```python
from build123d import *

# Parameters (mm, degrees)
SKETCH1_W           = 48.3
SKETCH1_H           = 45
SKETCH1_R           = 2.875
SKETCH1_R_2         = 1.25
SKETCH1_R_3         = 2.8
SKETCH1_R_4         = 2.5
BOSS_EXTRUDE1_DEPTH = 6.35


with BuildPart() as part:
    # Sketch1 → Boss-Extrude1 (new body)
    with BuildSketch(Plane(origin=(0, 0, 0), x_dir=(1, 0, 0), z_dir=(0, 1, 0))):
        with Locations((24.15, -22.5)):
            Rectangle(SKETCH1_W, SKETCH1_H)
        with Locations(Location((15.8, -12.5, 0), (0, 0, 270))):
            Circle(SKETCH1_R, mode=Mode.SUBTRACT)
        with Locations(Location((35.8, -12.5, 0), (0, 0, 270))):
            Circle(SKETCH1_R, mode=Mode.SUBTRACT)
        with Locations(Location((15.8, -32.5, 0), (0, 0, 270))):
            Circle(SKETCH1_R, mode=Mode.SUBTRACT)
        with Locations(Location((35.8, -32.5, 0), (0, 0, 270))):
            Circle(SKETCH1_R, mode=Mode.SUBTRACT)
        with Locations(Location((10.8, -7, 0), (0, 0, 270))):
            Circle(SKETCH1_R_2, mode=Mode.SUBTRACT)
        with Locations(Location((20.8, -7, 0), (0, 0, 270))):
            Circle(SKETCH1_R_2, mode=Mode.SUBTRACT)
        with Locations(Location((30.8, -7, 0), (0, 0, 270))):
            Circle(SKETCH1_R_2, mode=Mode.SUBTRACT)
        with Locations(Location((40.8, -7, 0), (0, 0, 270))):
            Circle(SKETCH1_R_2, mode=Mode.SUBTRACT)
        with Locations(Location((20.8, -17, 0), (0, 0, 270))):
            Circle(SKETCH1_R_2, mode=Mode.SUBTRACT)
        with Locations(Location((30.8, -17, 0), (0, 0, 270))):
            Circle(SKETCH1_R_2, mode=Mode.SUBTRACT)
        with Locations(Location((40.8, -17, 0), (0, 0, 270))):
            Circle(SKETCH1_R_2, mode=Mode.SUBTRACT)
        with Locations(Location((20.8, -27, 0), (0, 0, 270))):
            Circle(SKETCH1_R_2, mode=Mode.SUBTRACT)
        with Locations(Location((30.8, -27, 0), (0, 0, 270))):
            Circle(SKETCH1_R_2, mode=Mode.SUBTRACT)
        with Locations(Location((40.8, -27, 0), (0, 0, 270))):
            Circle(SKETCH1_R_2, mode=Mode.SUBTRACT)
        with Locations(Location((20.8, -37, 0), (0, 0, 270))):
            Circle(SKETCH1_R_2, mode=Mode.SUBTRACT)
        with Locations(Location((30.8, -37, 0), (0, 0, 270))):
            Circle(SKETCH1_R_2, mode=Mode.SUBTRACT)
        with Locations(Location((40.8, -37, 0), (0, 0, 270))):
            Circle(SKETCH1_R_2, mode=Mode.SUBTRACT)
        with Locations(Location((10.8, -17, 0), (0, 0, 270))):
            Circle(SKETCH1_R_2, mode=Mode.SUBTRACT)
        with Locations(Location((10.8, -27, 0), (0, 0, 270))):
            Circle(SKETCH1_R_2, mode=Mode.SUBTRACT)
        with Locations(Location((10.8, -37, 0), (0, 0, 270))):
            Circle(SKETCH1_R_2, mode=Mode.SUBTRACT)
        with Locations(Location((25.8, -12.5, 0), (0, 0, 270))):
            Circle(SKETCH1_R_3, mode=Mode.SUBTRACT)
        with Locations(Location((25.8, -32.5, 0), (0, 0, 270))):
            Circle(SKETCH1_R_3, mode=Mode.SUBTRACT)
        with Locations(Location((13.3, -22.5, 0), (0, 0, 270))):
            Circle(SKETCH1_R_4, mode=Mode.SUBTRACT)
        with Locations(Location((38.3, -22.5, 0), (0, 0, 270))):
            Circle(SKETCH1_R_4, mode=Mode.SUBTRACT)
    extrude(amount=BOSS_EXTRUDE1_DEPTH)


solid = part.part
```
Could you check a few things on this model? Use its own coordinates, in mm. Round coordinates to 2 decimals unless told otherwise and drop trailing zeros. Loops run counter-clockwise (first coordinate to the right, second up) from the corner with the lowest first, then second, coordinate; pieces in that order, holes last.
Q1. I want a section at D-D (z = 17). Write out the boundary of the cut face in (x, y).
Q2. I want a section at A-A (z = 24). Write out the boundary of the cut face in (x, y).
Q3. For P1, Ø5, axis at x = 25.8, z = 32.5, coming from the +Y side, with a flat end and sliding along its axis, tell me the tip position at first contact or that it passes through.
Q4. I want a section at C-C (y = 5.25). Give the number of separate pieces and of enclosed holes in the cut face, and give its area (3 significant figures).
Q5. Please list where these lines run through material, in increasing order: L1, parallel to X at y = 1.75, z = 12.5 (3 decimals); L2, parallel to X at y = 1.5, z = 34.5; L3, parallel to Z at x = 15, y = 2.5.
Q6. Thinking about a two-plate mould opening in Z: for faces 1 (the flat face through (24, 3, 45)), 2 (the cylindrical face through (37.74, 3.13, 30.38)), 3 (the flat face through (0, 3, 23)), 4 (the cylindrical face through (13.4, 3.1, 20)), which applies, pulls with the +Z half, pulls with the -Z half, needs draft (parallel to the pull), parting line crosses it, or undercut?
Q7. I want a section at B-B (z = 32.5). Write out the boundary of the cut face in (x, y) (3 decimals).
Answer below:
1. outline: (0, 0) - (9.55, 0) - (9.55, 6.35) - (0, 6.35) - close; (12.05, 0) - (19.55, 0) - (19.55, 6.35) - (12.05, 6.35) - close; (22.05, 0) - (29.55, 0) - (29.55, 6.35) - (22.05, 6.35) - close; (32.05, 0) - (39.55, 0) - (39.55, 6.35) - (32.05, 6.35) - close; (42.05, 0) - (48.3, 0) - (48.3, 6.35) - (42.05, 6.35) - close
2. outline: (0, 0) - (11.3, 0) - (11.3, 6.35) - (0, 6.35) - close; (15.3, 0) - (36.3, 0) - (36.3, 6.35) - (15.3, 6.35) - close; (40.3, 0) - (48.3, 0) - (48.3, 6.35) - (40.3, 6.35) - close
3. P1: passes through
4. separate pieces: 1
4. enclosed holes: 24
4. area: 1,900 mm2
5. L1: x = 0 to 12.925, 18.675 to 23, 28.6 to 32.925, 38.675 to 48.3
5. L2: x = 0 to 13.73, 17.87 to 23.84, 27.76 to 33.73, 37.87 to 48.3
5. L3: z = 0 to 9.74, 15.26 to 20.67, 24.33 to 29.74, 35.26 to 45
6. face 1: pulls with the +Z half
6. face 2: undercut
6. face 3: needs draft
6. face 4: undercut
7. outline: (0, 0) - (12.925, 0) - (12.925, 6.35) - (0, 6.35) - close; (18.675, 0) - (23, 0) - (23, 6.35) - (18.675, 6.35) - close; (28.6, 0) - (32.925, 0) - (32.925, 6.35) - (28.6, 6.35) - close; (38.675, 0) - (48.3, 0) - (48.3, 6.35) - (38.675, 6.35) - close
